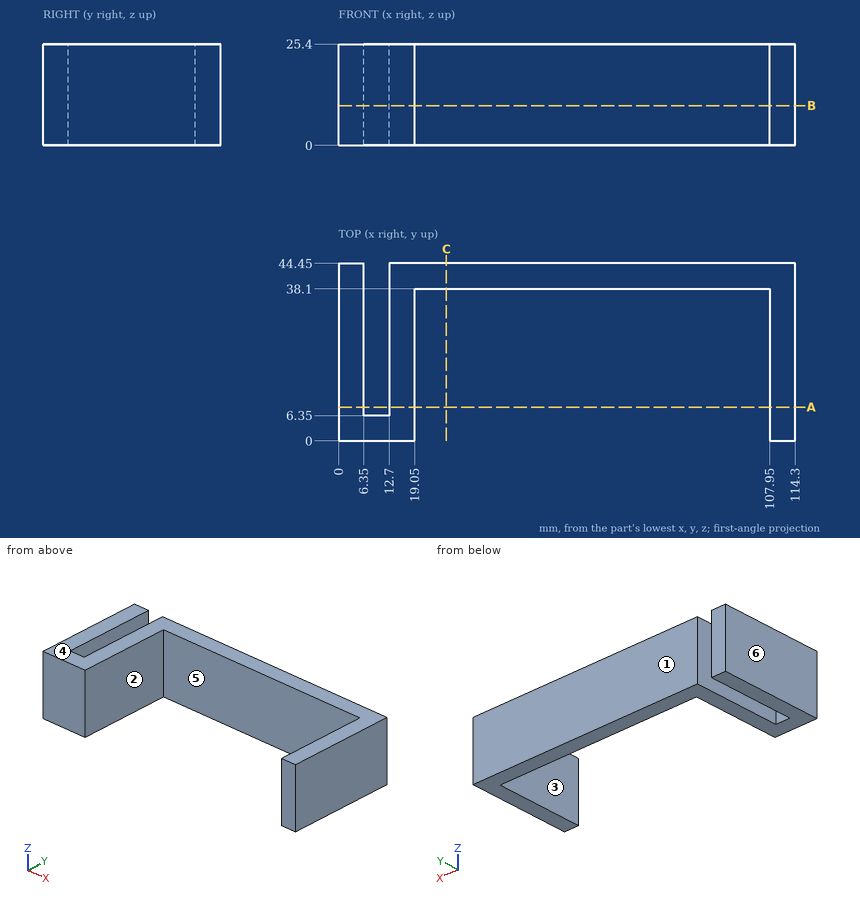
Can you work these out from the drawing? Everything is in mm from the part's minimum corner. A direction names the side the tool comes from. Round coordinates to 2 decimals unless told otherwise and drop trailing zeros. Order: outer loops, then holes, each group sorted by start corner. A loop starts at its lowest first (then second) coordinate and runs counter-clockwise, first axis right, second up. Notation, with made-up numbers: (-34.5, 80.25) -> (-20.5, 80.25) arc R25 ccw to (-20.5, 110.25) -> close; hole circle Ø10 at (57.25, -19). An arc over 180 degrees is marked (long way). Return JSON: item names as keys, results as strings. Group by question number.
1. If we section it at A-A, the plane y = 8.5: Write out the boundary of the cut face in (x, z), then the cut area to 3 significant figures.
2. I need wall thicknesses on line 1 (X direction, y = 38, z = 16.75); line 2 (X direction, y = 6, z = 2); line 3 (Y direction, x = 45.5, z = 15.5). Which ranges of each line are inside material? Lowest first, please. Write a range as [from, to].
3. We'd pull the mould along X, two halves only. Please class the marked faces 3, 4, 5 and 6: released by +X, released by -X, zero draft, split by the parting line, or undercut.
4. If we section it at C-C, the plane x = 27: Write out the boundary of the cut face in (y, z), then the cut area to 3 significant figures.
5. Which directions (+Z, -Z, +X, -X, +Y, -Y) give clear straight access to the entire face, cutting with the end or side of a thin tool? Please do the marked faces 1 and 2.
6. Will this pin go through, and if not, where does the flat tip stop? pin 1 (1.9 mm diameter, centred on x = 10.5, z = 16.5, fed in from +Y).
7. If we section it at B-B, the plane z = 10: Write out the boundary of the cut face in (x, y), then the cut area to 3 significant figures.
Output values:
{
 "1": {"outline": "(0, 0) -> (6.35, 0) -> (6.35, 25.4) -> (0, 25.4) -> close; (12.7, 0) -> (19.05, 0) -> (19.05, 25.4) -> (12.7, 25.4) -> close; (107.95, 0) -> (114.3, 0) -> (114.3, 25.4) -> (107.95, 25.4) -> close", "area": "484 mm²"},
 "2": {"line 1": "[0, 6.35], [12.7, 19.05], [107.95, 114.3]", "line 2": "[0, 19.05], [107.95, 114.3]", "line 3": "[38.1, 44.45]"},
 "3": {"face 3": "undercut", "face 4": "zero draft", "face 5": "undercut", "face 6": "released by -X"},
 "4": {"outline": "(38.1, 0) -> (44.45, 0) -> (44.45, 25.4) -> (38.1, 25.4) -> close", "area": "161 mm²"},
 "5": {"face 1": "+Z, -Z, +X, -X, +Y", "face 2": "+Z, -Z, -Y"},
 "6": {"pin 1": "y = 6.35"},
 "7": {"outline": "(0, 0) -> (19.05, 0) -> (19.05, 38.1) -> (107.95, 38.1) -> (107.95, 0) -> (114.3, 0) -> (114.3, 44.45) -> (12.7, 44.45) -> (12.7, 6.35) -> (6.35, 6.35) -> (6.35, 44.45) -> (0, 44.45) -> close", "area": "1,450 mm²"}
}
